Source: CAD feature listing. Evaluate the final solid. Frame: model axes, mm. A direction names the side the tool comes from. Give positions to 0.01 mm unless a question says otherwise; leave off trailing zeros. Write each loop counter-clockwise with the first axis right and the second up, starting at its lowest first coordinate (ties: lowest second). Pieces come first, ordered by that corner, then holes. Notation, with made-up numbers: (34, -9.75) -> (64, -9.75) arc R29 cw to (64, 10.25) -> close; hole circle Ø7 at (87, 15). An arc over 180 degrees is marked (long way). Answer as a JSON object with one key per item and string values. Group by question number.
Item 1: Access query for faces 5 (the face through (-25, 0, 14)), 6 (the face through (0, -22, 14)). Directions: +Z, -Z, +X, -X, +Y, -Y. A direction counts if a zero-diameter tool reaches every point of the face in a straight line with its end or side. Return the directions, or none.
Item 2: Section query A-A on y = -8.5. Return the cut outline in (x, z), plus the area to 3 significant figures.
Item 3: Pull-direction query (Y, two-part tool) for faces 1 (the face through (-22, 0, 14)), 2 (the face through (0, -25, 14)), 3 (the face through (0, 25, 13)), 4 (the face through (22, 0, 14)); classes: pulls with the +Y half, pulls with the -Y half, needs draft (parallel to the pull), parting line crosses it, or undercut.
Item 4: Ray query, probe 1 along Y at (x, z) = (13, 122); probe 2 along Y at (x, z) = (21, 534). Return the intervals inside material, ascending. Write a range as from..to.
Item 5: Section query B-B on x = -2. Return the cut outline in (y, z).
Item 6: Section query C-C on z = -474. Return the cut outline in (x, y).
from build123d import *

# Parameters (mm, degrees)
F1_DEPTH      = 1000
F3_DEPTH      = 2000.001
F5_DEPTH      = 25.001
F5_DEPTH_BACK = 25


# Not quite as in the source:
# - a pattern or mirror of a feature is missing from the dataset's text; its kind, count and spacing are read off the source's solid


with BuildPart() as f1:
    # F0 (on Top) → F1 (new body, symmetric)
    with BuildSketch(Plane.XY):
        with BuildLine():
            ThreePointArc((25, 20), (23.5355339059, 23.5355339059), (20, 25))
            Line((20, 25), (-20, 25))
            ThreePointArc((-20, 25), (-23.5355339059, 23.5355339059), (-25, 20))
            Line((-25, 20), (-25, -20))
            ThreePointArc((-25, -20), (-23.5355339059, -23.5355339059), (-20, -25))
            Line((-20, -25), (20, -25))
            ThreePointArc((20, -25), (23.5355339059, -23.5355339059), (25, -20))
            Line((25, -20), (25, 20))
        make_face()
    extrude(amount=F1_DEPTH, both=True)

    # F2 (on face) → F3 (cut, through all)
    with BuildSketch(Plane.XY.offset(1000)):
        with BuildLine():
            ThreePointArc((-22, -20), (-21.4142135624, -21.4142135624), (-20, -22))
            Line((-20, -22), (20, -22))
            ThreePointArc((20, -22), (21.4142135624, -21.4142135624), (22, -20))
            Line((22, -20), (22, 20))
            ThreePointArc((22, 20), (21.4142135624, 21.4142135624), (20, 22))
            Line((20, 22), (-20, 22))
            ThreePointArc((-20, 22), (-21.4142135624, 21.4142135624), (-22, 20))
            Line((-22, 20), (-22, -20))
        make_face()
    extrude(amount=-F3_DEPTH, mode=Mode.SUBTRACT)

    # F4 (on Right) → F5 (cut, two sides)
    with BuildSketch(Plane.YZ) as f5_sk:
        Polygon((25, 1000), (-25, 1000), (25, 950), align=None)
    f5 = extrude(amount=-F5_DEPTH, mode=Mode.SUBTRACT) + extrude(f5_sk.sketch, amount=F5_DEPTH_BACK, mode=Mode.SUBTRACT)

    # F5_copies: F5 across plane
    add(f5.mirror(Plane(origin=(0, 0, 0), x_dir=(-1, 0, 0), z_dir=(0, 0, -1))), mode=Mode.SUBTRACT)


solid = f1.part
Worked answers:
{
 "1": {"face 5": "+Z, -Z, -X, +Y, -Y", "face 6": "+Z, -Z"},
 "2": {"outline": "(-25, -983.5) -> (-22, -983.5) -> (-22, 983.5) -> (-25, 983.5) -> close; (22, -983.5) -> (25, -983.5) -> (25, 983.5) -> (22, 983.5) -> close", "area": "11,800 mm^2"},
 "3": {"face 1": "undercut", "face 2": "pulls with the -Y half", "face 3": "pulls with the +Y half", "face 4": "undercut"},
 "4": {"probe 1": "-25..-22, 22..25", "probe 2": "-24.9..-21.73, 21.73..24.9"},
 "5": {"outline": "(-25, -1000) -> (-22, -997) -> (-22, 997) -> (-25, 1000) -> close; (22, -953) -> (25, -950) -> (25, 950) -> (22, 953) -> close"},
 "6": {"outline": "(-25, -20) arc R5 ccw to (-20, -25) -> (20, -25) arc R5 ccw to (25, -20) -> (25, 20) arc R5 ccw to (20, 25) -> (-20, 25) arc R5 ccw to (-25, 20) -> close; hole (-22, -20) arc R2 ccw to (-20, -22) -> (20, -22) arc R2 ccw to (22, -20) -> (22, 20) arc R2 ccw to (20, 22) -> (-20, 22) arc R2 ccw to (-22, 20) -> close"}
}
